Can you work these out from the model? Positions are in its coordinate system, mm. Face numbers are marked on the shaded views. A direction names the side the tool comes from. Coordinates: 2 decimals unless noted, no trailing zeros. Order: outer loops, then holes, each group sorted by start corner. A loop starts at its lowest first (then second) coordinate and runs counter-clockwise, first axis right, second up. Notation, with made-up numbers: (87.5, 12) -> (105.5, 12) arc R25 ccw to (105.5, 25) -> close; hole circle Ø3 at (38, 28). An arc over 180 degrees is marked (long way). Answer as a JSON object with one key per item and string values. Group by question number.
(1) I want a section at A-A, the plane z = -9.75. List the corners of the cut face in (x, y) for me.
(2) For pin 1 (4 mm diameter, centred on x = -5, y = 15, fed in from +Z), with a flat end and sliding along its axis, tell me the tip position at first contact or that it passes through.
(3) If we mould it in two halves opening along X, with no side actions, what happens to the marked faces 3, 4 and 5? For each: pulls with the +X half, pulls with the -X half, needs draft (parallel to the pull), parting line crosses it, or undercut.
(4) Which directions (+Z, -Z, +X, -X, +Y, -Y) give clear straight access to the entire face, cutting with the end or side of a thin tool? Please do the marked faces 1 and 2.
(5) I need wall thicknesses on line 1 (X direction, y = 25, z = -15); line 2 (Z direction, x = -7, y = 26); line 3 (Y direction, x = -14, z = 0.25). Which ranges of each line are inside material? Lowest first, please.
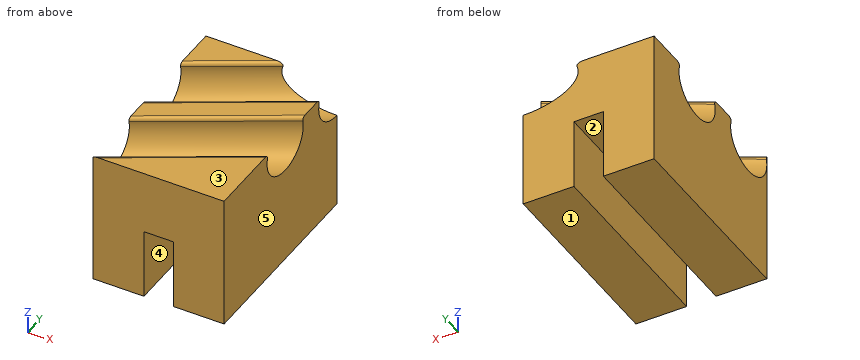
from build123d import *

# Parameters (mm, degrees)
F1_DEPTH      = 24
F1_DEPTH_BACK = 1.5
F4_T1_DEPTH   = 17.3810892057
F4_T3_DEPTH   = 26.4408905281
F4_T5_DEPTH   = 26.4408905281
F4_T7_DEPTH   = 26.4408905281
F6_DEPTH      = 43.7
F7_DEPTH      = 5


# Not quite as in the source:
# - a fillet or chamfer that OpenCascade refuses, or shapes differently, is made with other operations: its cross-section is extruded or revolved along the edge and cut away or added
# - a feature names something its author has since deleted; it is built from what else it names


with BuildPart() as f1:
    # F0 (on Top) → F1 (new body, two sides)
    with BuildSketch(Plane.XY) as f1_sk:
        Polygon((-9.9499136187, 28.9028368274), (-21.5499136187, 28.9028368274), (-21.5499136187, 22.2055737048), align=None)
        Polygon((-1.5499136187, 28.9028368274), (-9.9499136187, 28.9028368274), (-21.5499136187, 22.2055737048), (-21.5499136187, 17.3558314436), align=None)
        Polygon((-1.5499136187, 21.9746335971), (-1.5499136187, 28.9028368274), (-21.5499136187, 17.3558314436), (-21.5499136187, 10.4276282133), align=None)
        Polygon((-1.5499136187, 15.0464303668), (-1.5499136187, 21.9746335971), (-21.5499136187, 10.4276282133), (-21.5499136187, 3.499424983), align=None)
        Polygon((-1.5499136187, -1.3503172782), (-1.5499136187, 10.1966881056), (-21.5499136187, -1.3503172782), align=None)
        Polygon((-1.5499136187, 10.1966881056), (-1.5499136187, 15.0464303668), (-21.5499136187, 3.499424983), (-21.5499136187, -1.3503172782), align=None)
    extrude(amount=-F1_DEPTH)
    extrude(f1_sk.sketch, amount=F1_DEPTH_BACK)

    # F0 (on Top) → F2 (revolve, cut)
    with BuildSketch(Plane.XY):
        Polygon((-21.5499136187, 17.3558314436), (-21.5499136187, 22.2055737048), (-34.8505816362, 14.5264294445), (-32.7505816362, 10.8891227486), align=None)
        Polygon((-1.5499136187, 28.9028368274), (-9.9499136187, 28.9028368274), (-21.5499136187, 22.2055737048), (-21.5499136187, 17.3558314436), align=None)
        Polygon((0, 34.6474221335), (-9.9499136187, 28.9028368274), (-1.5499136187, 28.9028368274), (2.1, 31.0101154376), align=None)
    revolve(axis=Axis((-15.3252908181, 20.9496190931, 0), (-0.8660254038, -0.5, 0)), mode=Mode.SUBTRACT)

    # F0 (on Top) → F3 (revolve, cut)
    with BuildSketch(Plane.XY):
        Polygon((-21.5499136187, -1.3503172782), (-21.5499136187, 3.499424983), (-26.7505816362, 0.4968179032), (-24.6505816362, -3.1404887927), align=None)
        Polygon((-1.5499136187, 10.1966881056), (-1.5499136187, 15.0464303668), (-21.5499136187, 3.499424983), (-21.5499136187, -1.3503172782), align=None)
        Polygon((8.1, 20.6178105922), (-1.5499136187, 15.0464303668), (-1.5499136187, 10.1966881056), (10.2, 16.9805038963), align=None)
    revolve(axis=Axis((-9.3252908181, 10.5573142477, 0), (-0.8660254038, -0.5, 0)), mode=Mode.SUBTRACT)

    # F4: fillet of radius 0.5 on 4 edges, made by hand

    # F4_s2 → F4_t1 (cut)
    with BuildSketch(Plane(origin=(6.9175881272, 3.9938713674, 0), x_dir=(0, 0, 1), z_dir=(-0.8660254038, -0.5, 0))):
        with BuildLine():
            ThreePointArc((1.5, 30.3979327446), (1.3136945255, 30.0085797625), (0.8936170213, 29.9093811487))
            ThreePointArc((0.8936170213, 29.9093811487), (1.2002187189, 29.8304048869), (1.5, 29.7285567925))
            Line((1.5, 29.7285567925), (1.5, 30.3979327446))
        make_face()
    extrude(amount=F4_T1_DEPTH, mode=Mode.SUBTRACT)

    # F4_s4 → F4_t3 (cut)
    with BuildSketch(Plane(origin=(10.8405971764, 6.258821698, 0), x_dir=(0, 0, 1), z_dir=(-0.8660254038, -0.5, 0))):
        with BuildLine():
            ThreePointArc((0.8936170213, 21.7017143379), (1.3136945255, 21.6025157241), (1.5, 21.213162742))
            Line((1.5, 21.213162742), (1.5, 21.8825386941))
            ThreePointArc((1.5, 21.8825386941), (1.2002187189, 21.7806905996), (0.8936170213, 21.7017143379))
        make_face()
    extrude(amount=F4_T3_DEPTH, mode=Mode.SUBTRACT)

    # F4_s6 → F4_t5 (cut)
    with BuildSketch(Plane(origin=(-14.1348766704, -8.1607748506, 0), x_dir=(0, 0, 1), z_dir=(0.8660254038, 0.5, 0))):
        with BuildLine():
            ThreePointArc((1.5, -18.3979327446), (1.3136945255, -18.0085797625), (0.8936170213, -17.9093811487))
            ThreePointArc((0.8936170213, -17.9093811487), (1.2002187189, -17.8304048869), (1.5, -17.7285567925))
            Line((1.5, -17.7285567925), (1.5, -18.3979327446))
        make_face()
    extrude(amount=F4_T5_DEPTH, mode=Mode.SUBTRACT)

    # F4_s8 → F4_t7 (cut)
    with BuildSketch(Plane(origin=(-18.0578857196, -10.4257251812, 0), x_dir=(0, 0, 1), z_dir=(0.8660254038, 0.5, 0))):
        with BuildLine():
            ThreePointArc((0.8936170213, -9.7017143379), (1.3136945255, -9.6025157241), (1.5, -9.213162742))
            Line((1.5, -9.213162742), (1.5, -9.8825386941))
            ThreePointArc((1.5, -9.8825386941), (1.2002187189, -9.7806905996), (0.8936170213, -9.7017143379))
        make_face()
    extrude(amount=F4_T7_DEPTH, mode=Mode.SUBTRACT)

    # F5 (on face) → F6 (cut)
    with BuildSketch(Plane.XZ.offset(1.3503172782)):
        Polygon((-13.7999136187, -26.7), (-9.2999136187, -26.7), (-9.8499136187, -24), (-13.2499136187, -24), align=None)
        Polygon((-9.8499136187, -24), (-9.2999136187, -24), (-9.2999136187, -8.2), (-13.7999136187, -8.2), (-13.7999136187, -24), (-13.2499136187, -24), align=None)
    extrude(amount=-F6_DEPTH, mode=Mode.SUBTRACT)

    # F7 (cut): faces of the model
    f7_faces = [f1.faces().sort_by_distance(p)[0] for p in [
        (-17.6749136187, 13.7762597746, -24),
        (-5.4249136187, 13.7762597746, -24),
    ]]
    extrude(f7_faces, amount=-F7_DEPTH, mode=Mode.SUBTRACT)


solid = f1.part
Computed values:
{
 "1": {"outline": "(-21.55, -1.35) -> (-13.8, -1.35) -> (-13.8, 28.9) -> (-21.55, 28.9) -> close; (-9.3, -1.35) -> (-1.55, -1.35) -> (-1.55, 28.9) -> (-9.3, 28.9) -> close"},
 "2": {"pin 1": "stops at z = -2.02"},
 "3": {"face 3": "needs draft", "face 4": "undercut", "face 5": "pulls with the +X half"},
 "4": {"face 1": "-Z, +X, -X, +Y, -Y", "face 2": "-Z, +Y, -Y"},
 "5": {"line 1": "x = -21.55 to -13.8, -9.3 to -1.55", "line 2": "z = -19 to -4.19", "line 3": "y = -1.35 to 3.02, 12.7 to 16.87, 26.56 to 28.9"}
}
